Input: dimensioned drawing with shaded views. Units: mm. Origin: part minimum x, y, z. A direction names the side the tool comes from. Coordinates: 2 decimals unless noted, no trailing zeros. Order: outer loops, then holes, each group sorted by start corner. A loop starts at its lowest first (then second) coordinate and runs counter-clockwise, first axis right, second up.
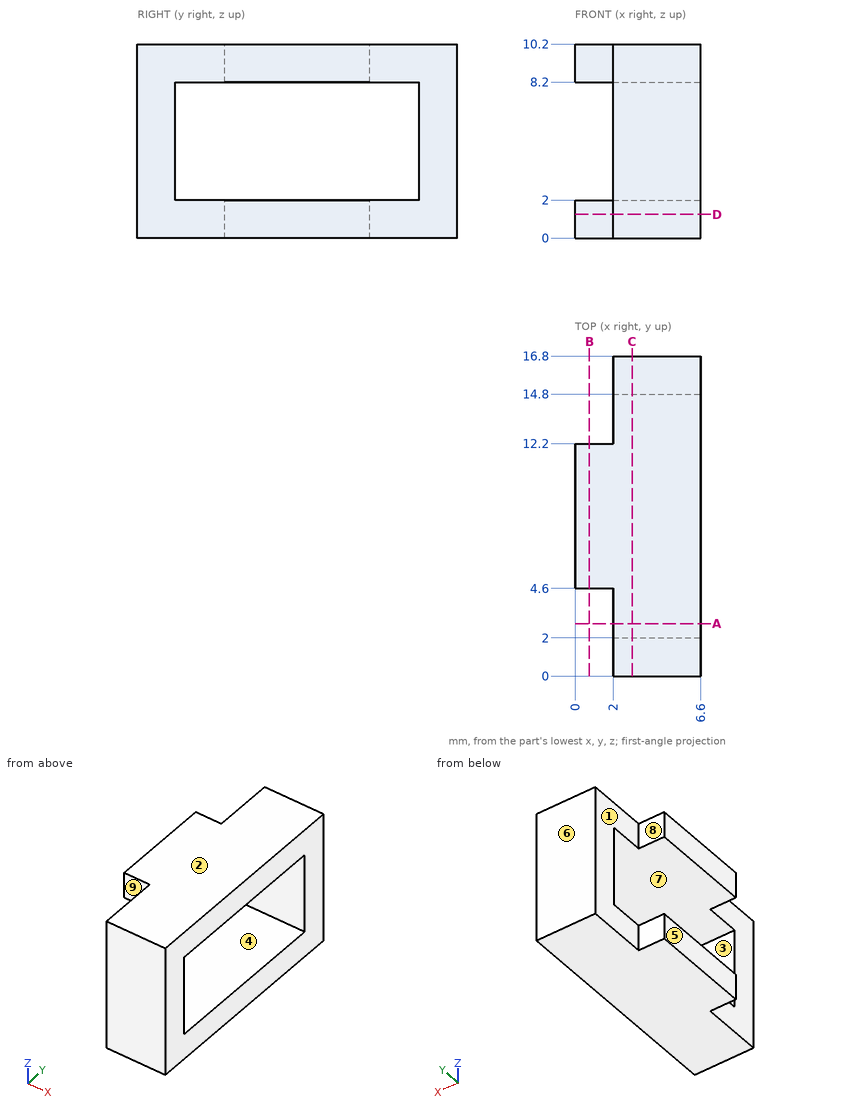
1. Draft query along Z for the marked faces 1, 2, 3 and 4. Return one class per face: released by +Z, released by -Z, zero draft, split by the parting line, or undercut.
Findings:
face 1: zero draft
face 2: released by +Z
face 3: undercut
face 4: undercut
2. Section query B-B on x = 0.75. Return loops of the section in (y, z).
Findings:
outline: (4.6, 0) - (12.2, 0) - (12.2, 2) - (4.6, 2) - close; (4.6, 8.2) - (12.2, 8.2) - (12.2, 10.2) - (4.6, 10.2) - close
3. Access query for the marked faces 5, 6, 7, 8 and 9. Directions: +Z, -Z, +X, -X, +Y, -Y. A direction counts if a zero-diameter tool reaches every point of the face in a straight line with its end or side. Return the directions, or none.
Findings:
face 5: +Z, -Z, -X, +Y, -Y
face 6: +Z, -Z, +X, -X, +Y
face 7: +X, -X
face 8: +Z, -Z, -X, +Y
face 9: +Z, -Z, -X, -Y
4. Pin query (flat end, axial travel): P1, Ø0.6, axis at x = 1, z = 1, coming from the -Y side; P2, Ø5, axis at y = 1.5, z = 4, coming from the -X side; P3, Ø3, axis at y = 12, z = 4.5, coming from the -X side; P4, Ø1, axis at x = 1, z = 0.5, coming from the +Y side. Return the tip coordinate at first contact, or that it passes through.
Findings:
P1: stops at y = 4.6
P2: stops at x = 2
P3: passes through
P4: stops at y = 12.2
5. Section query A-A on y = 2.75. Return loops of the section in (x, z), plus the area to 3 significant figures.
Findings:
outline: (2, 0) - (6.6, 0) - (6.6, 2) - (2, 2) - close; (2, 8.2) - (6.6, 8.2) - (6.6, 10.2) - (2, 10.2) - close
area: 18.4 mm2
6. Section query D-D on z = 1.25. Return loops of the section in (x, y), plus the area to 3 significant figures.
Findings:
outline: (0, 4.6) - (2, 4.6) - (2, 0) - (6.6, 0) - (6.6, 16.8) - (2, 16.8) - (2, 12.2) - (0, 12.2) - close
area: 92.5 mm2
7. Ray query, line 1 (Y direction, x = 5.5, z = 3.5); line 2 (Z direction, x = 0.5, y = 5.5); line 3 (X direction, y = 15.25, z = 1.75). Return the intervals inside material, ascending.
Findings:
line 1: y = 0 to 2, 14.8 to 16.8
line 2: z = 0 to 2, 8.2 to 10.2
line 3: x = 2 to 6.6
8. Section query C-C on x = 3. Return loops of the section in (y, z).
Findings:
outline: (0, 0) - (16.8, 0) - (16.8, 10.2) - (0, 10.2) - close; hole (2, 2) - (14.8, 2) - (14.8, 8.2) - (2, 8.2) - close
